Build history of the part. All positions in model axes, mm. Round coordinates to 2 decimals unless told otherwise and drop trailing zeros. Loops run counter-clockwise (first coordinate to the right, second up) from the corner with the lowest first, then second, coordinate; pieces in that order, holes last. Notation, with made-up numbers: (-14.5, 58) -> (-8.5, 58) arc R22 ccw to (-8.5, 95) -> close; hole circle Ø9 at (-0.75, 46). An arc over 180 degrees is marked (long way). Put each result on its own line as item: value. Start each with the question number.
```python
from build123d import *

# Parameters (mm, degrees)
F1_W     = 6
F1_H     = 3
F1_W_2   = 12
F2_DEPTH = 3


with BuildPart() as f2:
    # F1 (on Front) → F2 (new body)
    with BuildSketch(Plane.XZ):
        Polygon((-49, 75), (49, 75), (0, 124), align=None)
        with BuildLine():
            Line((43, -75), (49, -75))
            Line((49, -75), (49, 0))
            ThreePointArc((49, 0), (47, 37.5), (49, 75))
            Line((49, 75), (-49, 75))
            ThreePointArc((-49, 75), (-47, 37.5), (-49, 0))
            Line((-49, 0), (-49, -75))
            Line((-49, -75), (-43, -75))
            Line((-43, -75), (-43, 0))
            Line((-43, 0), (-40, 0))
            Line((-40, 0), (-40, -75))
            Line((-40, -75), (-28, -75))
            Line((-28, -75), (28, -75))
            Line((28, -75), (40, -75))
            Line((40, -75), (40, 0))
            Line((40, 0), (43, 0))
            Line((43, 0), (43, -75))
        make_face()
        with Locations((-46, -76.5)):
            Rectangle(F1_W, F1_H)
        with Locations((-34, -76.5)):
            Rectangle(F1_W_2, F1_H)
        with Locations((34, -76.5)):
            Rectangle(F1_W_2, F1_H)
        with Locations((46, -76.5)):
            Rectangle(F1_W, F1_H)
        with BuildLine():
            Line((-49, -75), (-49, 0))
            ThreePointArc((-49, 0), (-51, -37.5), (-49, -75))
        make_face()
        with BuildLine():
            Line((49, 0), (49, -75))
            ThreePointArc((49, -75), (51, -37.5), (49, 0))
        make_face()
    extrude(amount=F2_DEPTH)


solid = f2.part
```
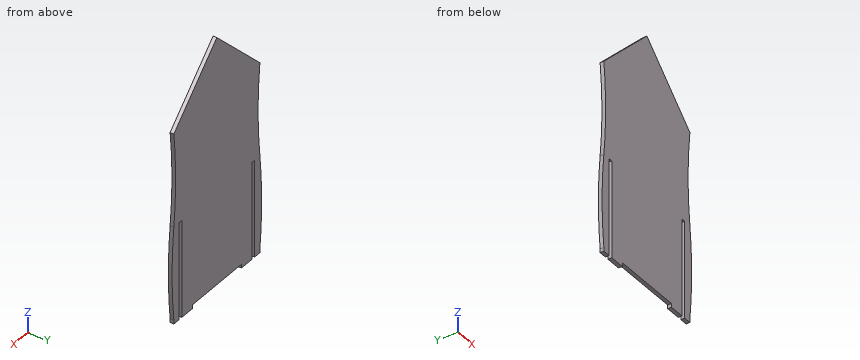
Item 1: Cut at A-A on z = -37.5. Write the cut outline in (x, y), then the cut area to 3 significant figures.
Item 2: Cut at D-D on z = -60.5. Write the cut outline in (x, y).
Item 3: Drop flat-ended pins along their axis: pin 1 (0.9 mm diameter, centred on x = -4.5, y = -1.5, fed in from -Z); pin 2 (1.5 mm diameter, centred on x = -41, y = -2, fed in from -Z); pin 3 (1.5 mm diameter, centred on y = -1, z = -76, fed in from +X). Give the stop position or say it passes through.
Item 4: Cut at B-B on y = -2.55. Write the cut outline in (x, z) (1 decimal), then the cut area to 3 significant figures.
Item 5: Cut at C-C on x = 21.5. Write the cut outline in (y, z).
Item 6: Wall check: line 1 (X direction, y = -0.85, z = -18.5); line 2 (X direction, y = -2, z = -54); line 3 (Z direction, x = 36, y = -2.55). Give the ranges that are in metal, low to high. Write a range as from..to.
Ans:
1. outline: (-51, -3) -> (-43, -3) -> (-43, 0) -> (-51, 0) -> close; (-40, -3) -> (40, -3) -> (40, 0) -> (-40, 0) -> close; (43, -3) -> (51, -3) -> (51, 0) -> (43, 0) -> close
1. area: 288 mm2
2. outline: (-50.25, -3) -> (-43, -3) -> (-43, 0) -> (-50.25, 0) -> close; (-40, -3) -> (40, -3) -> (40, 0) -> (-40, 0) -> close; (43, -3) -> (50.25, -3) -> (50.25, 0) -> (43, 0) -> close
3. pin 1: stops at z = -75
3. pin 2: stops at z = 0
3. pin 3: stops at x = 49
4. outline: (-49, -78) -> (-43, -78) -> (-43, 0) -> (-40, 0) -> (-40, -78) -> (-28, -78) -> (-28, -75) -> (28, -75) -> (28, -78) -> (40, -78) -> (40, 0) -> (43, 0) -> (43, -78) -> (49, -78) -> (49, -75) arc R352.6 ccw to (49, 0) arc R352.6 cw to (49, 75) -> (0, 124) -> (-49, 75) arc R352.6 cw to (-49, 0) arc R352.6 ccw to (-49, -75) -> close
4. area: 16,800 mm2
5. outline: (-3, -75) -> (0, -75) -> (0, 102.5) -> (-3, 102.5) -> close
6. line 1: x = -50.49..-43, -40..40, 43..50.49
6. line 2: x = -50.61..-43, -40..40, 43..50.61
6. line 3: z = -78..88
